Verification items for the finished model (mm, model axes). Face numbers are marked on the shaded views. A direction names the side the tool comes from. Round coordinates to 2 decimals unless told otherwise and drop trailing zeros. Write each loop counter-clockwise with the first axis right and the second up, starting at its lowest first coordinate (ties: lowest second). Pieces come first, ordered by that corner, then holes. Notation, with made-up numbers: M -36,-20.5 L 9,-20.5 A18 ccw 9,2.5 Z; hole C 3,50.5 d8. An arc over 180 degrees is marked long. Answer in a Markdown table with one row per item. Add a question column.
1. Go/stop test with flat-tipped pins: pin 1 Ø1 at (y, z) = (1.5, -1.5) entering from -X; pin 2 Ø5 at (y, z) = (-7, -2) entering from -X; pin 3 Ø5 at (x, z) = (-7.5, 1.5) entering from +Y. Record where each tip stops, or that it passes through.
2. Sectioned sample at B-B on x = -1.5. Record the cut outline in (y, z), plus the area to 3 significant figures.
3. Sectioned sample at C-C on y = -14. Record the cut outline in (x, z), plus the area to 3 significant figures.
4. Draft check along Y on the marked faces 1, 2, 3 and 4. Enter one of: pulls with the +Y half, pulls with the -Y half, needs draft (parallel to the pull), parting line crosses it, or undercut.
5. Material ranges on probe 1 along X at (y, z) = (-13.5, -1.75); probe 2 along Y at (x, z) = (-3.5, 3.75); probe 3 along X at (y, z) = (-12, 0), recorded low to high.
6. Set-up check for the marked faces 5, 6 and 7: record each of +Z, -Z, +X, -X, +Y, -Y from which the full face is reachable in a straight line by a thin tool's end or side.
7. Sectioned sample at D-D on x = -5.75. Record the cut outline in (y, z).
```python
from build123d import *

# Parameters (mm, degrees)
F1_DEPTH    = 5
F2_R        = 2
F3_R        = 0.99999
F4_T1_DEPTH = 18.321255839


# Not quite as in the source:
# - a fillet or chamfer that OpenCascade refuses, or shapes differently, is made with other operations: its cross-section is extruded or revolved along the edge and cut away or added
# - a fillet or chamfer is up to 0.001 mm smaller than in the source, because OpenCascade refuses the exact size


with BuildPart() as f1:
    # F0 (on Top) → F1 (new body, symmetric)
    with BuildSketch(Plane.XY):
        Polygon((-3.2426406871, -26.7513532198), (1, -22.5087125327), (1, 4.8656561381), (0, 4.8656561381), (-1, -10.1343438619), (-11.3743686708, -10.1343438619), (-15.6170093579, -14.3769845491), (-14.2027957955, -14.3769845491), (-10.6672618896, -10.8414506431), (0.2928932188, -21.8016057515), (-3.2426406871, -25.3371396575), align=None)
        Polygon((-3.9497474683, -27.458460001), (-3.2426406871, -26.7513532198), (-4.6568542495, -26.7513532198), align=None)
        Polygon((-4.6568542495, -26.7513532198), (-3.2426406871, -26.7513532198), (-3.2426406871, -25.3371396575), align=None)
        Polygon((-4.6568542495, -25.3371396575), (-4.6568542495, -26.7513532198), (-3.2426406871, -25.3371396575), align=None)
        Polygon((-15.6170093579, -15.7911981114), (-15.6170093579, -14.3769845491), (-16.3241161391, -15.0840913303), align=None)
        Polygon((-14.2027957955, -14.3769845491), (-15.6170093579, -14.3769845491), (-15.6170093579, -15.7911981114), align=None)
        Polygon((-14.2027957955, -15.7911981114), (-14.2027957955, -14.3769845491), (-15.6170093579, -15.7911981114), align=None)
    extrude(amount=F1_DEPTH, both=True)

    # F2
    f2_edges = [f1.edges().sort_by_distance(p)[0] for p in [
        (-11.374369, -10.134344, 0),
        (1, -22.508713, 0),
    ]]
    fillet(f2_edges, radius=F2_R)

    # F3 (radius 1 in the source; OpenCascade refuses exactly that, so slightly less here)
    f3_edges = [f1.edges().sort_by_distance(p)[0] for p in [
        (-16.324116, -15.084091, 0),
        (-3.949747, -27.45846, 0),
    ]]
    fillet(f3_edges, radius=F3_R)

    # F4: fillet of radius 2 on 1 edges, made by hand

    # F4_s2 → F4_t1 (cut)
    with BuildSketch(Plane.XY.offset(-9.1606279195)):
        with BuildLine():
            ThreePointArc((1, 4.8656561381), (0.2224588554, 4.1839894082), (-0.1107043409, 3.2050910239))
            Line((-0.1107043409, 3.2050910239), (0, 4.8656561381))
            Line((0, 4.8656561381), (1, 4.8656561381))
        make_face()
    extrude(amount=F4_T1_DEPTH, mode=Mode.SUBTRACT)


solid = f1.part
```
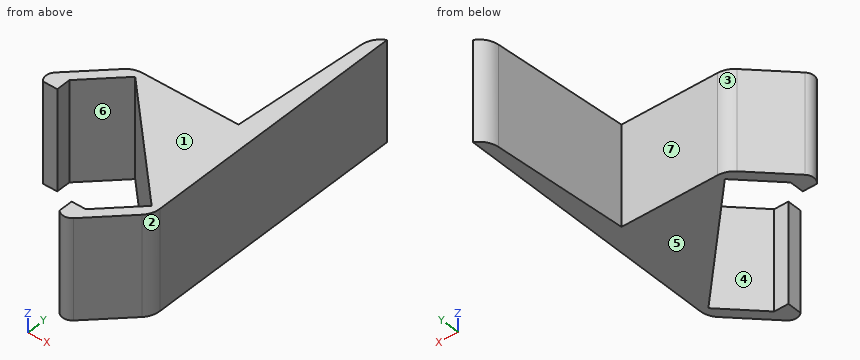
Geometry check:
| question | item | result |
|---|---|---|
| 1 | pin 1 | stops at x = -0.26 |
| 1 | pin 2 | stops at x = -0.96 |
| 1 | pin 3 | stops at y = -10.13 |
| 2 | outline | M -25.01,-5 L -23.59,-5 L -23.59,5 L -25.01,5 Z; M -20.01,-5 L -10.13,-5 L -10.13,5 L -20.01,5 Z |
| 2 | area | 113 mm2 |
| 3 | outline | M -15.24,-5 L -13.83,-5 L -13.83,5 L -15.24,5 Z; M -7.51,-5 L 1,-5 L 1,5 L -7.51,5 Z |
| 3 | area | 99.2 mm2 |
| 4 | face 1 | needs draft |
| 4 | face 2 | pulls with the -Y half |
| 4 | face 3 | pulls with the +Y half |
| 4 | face 4 | undercut |
| 5 | probe 1 | x = -14.74 to -13.33, -8.01 to 1 |
| 5 | probe 2 | y = -26.94 to -25.34, -18.01 to -10.13 |
| 5 | probe 3 | x = -13.24 to -11.83, -9.51 to 1 |
| 6 | face 5 | -Z, +X, -X, +Y, -Y |
| 6 | face 6 | +Z, -Z, -Y |
| 6 | face 7 | +Z, -Z, -X, +Y |
| 7 | outline | M -15.76,-5 L -10.13,-5 L -10.13,5 L -15.76,5 Z |
